Source: three-view drawing plus pictorial views. Frame: mm from the lowest corner of the part. A direction names the side the tool comes from. Round coordinates to 2 decimals unless told otherwise and drop trailing zeros. Loops run counter-clockwise (first coordinate to the right, second up) from the corner with the lowest first, then second, coordinate; pieces in that order, holes last. Notation, with made-up numbers: (2.25, 68.25) -> (32.25, 68.25) arc R8 ccw to (32.25, 80.25) -> close; hole circle Ø5 at (88, -34.75). An arc over 180 degrees is marked (long way). One line per question, with ' | ' between items. Start each with the question number.
Q1. Material intervals for L1, parallel to X at y = 1.25, z = 7.02; L2, parallel to X at y = 1, z = 1.94 (1 decimal); L3, parallel to X at y = 0.3, z = 2.75, sorted ascending.
Q2. Cut plane B-B on z = 8.75. Return loops of the section in (x, y).
Q3. Cut plane D-D on z = 5.75. Return loops of the section in (x, y).
Q4. Cut plane C-C on y = 1.15. Return loops of the section in (x, z), and give its area (3 significant figures).
Q5. Contact query for flat-ended pins moving along their axis: P1, Ø4, axis at x = 2.06, z = 8.75, coming from the -Y side; P2, Ø1, axis at x = 4.5, z = 3.5, coming from the +Y side. Output: stop coordinate, or through.
Q6. Cut plane A-A on x = 15. Return loops of the section in (y, z).
Q7. Mould query, pull axis X, two halves, no side actions, for the marked faces 1, 2 and 3. Classes: pulls with the +X half, pulls with the -X half, needs draft (parallel to the pull), parting line crosses it, or undercut.
Q8. Access query for the marked faces 4 and 5. Directions: +Z, -Z, +X, -X, +Y, -Y. A direction counts if a zero-diameter tool reaches every point of the face in a straight line with its end or side. Return the directions, or none.
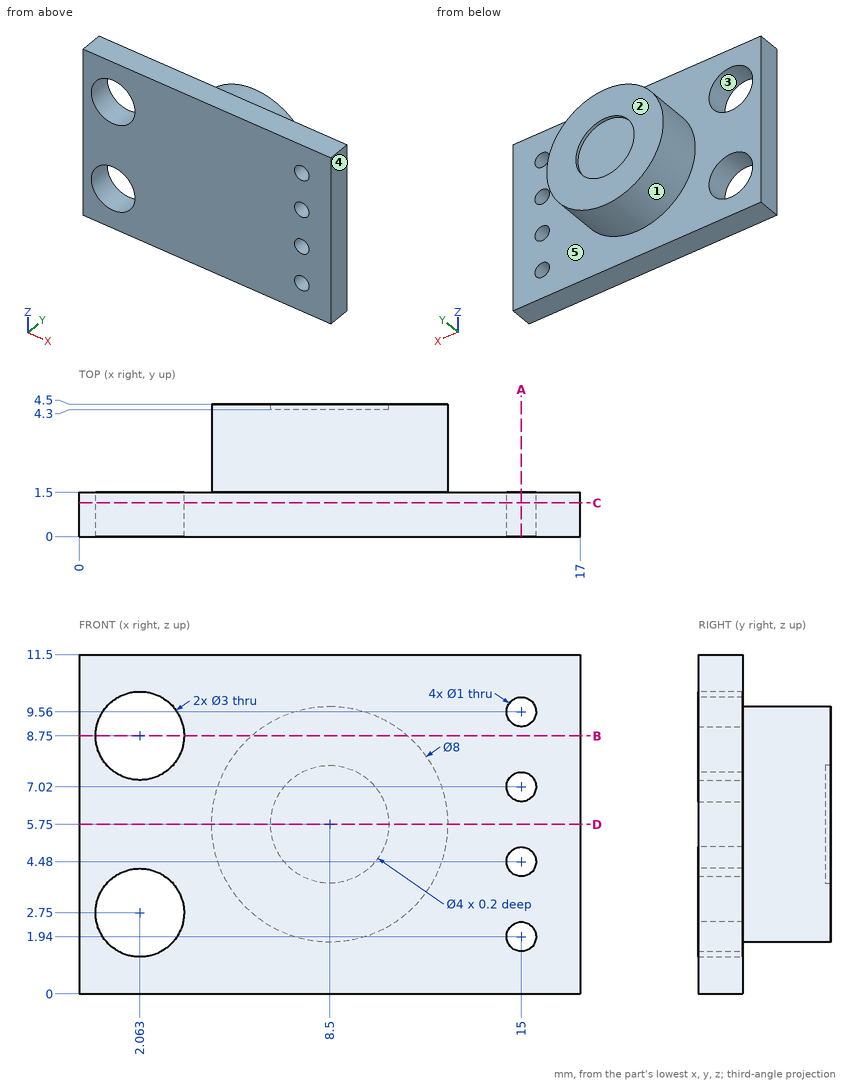
Results:
1) L1: 0 to 14.5, 15.5 to 17 | L2: 0 to 0.8, 3.3 to 14.5, 15.5 to 17 | L3: 0 to 0.56, 3.56 to 17
2) outline: (0, 0) -> (0.56, 0) -> (0.56, 1.5) -> (0, 1.5) -> close; (3.56, 0) -> (17, 0) -> (17, 1.5) -> (11.15, 1.5) -> (11.15, 4.5) -> (5.85, 4.5) -> (5.85, 1.5) -> (3.56, 1.5) -> close
3) outline: (0, 0) -> (17, 0) -> (17, 1.5) -> (12.5, 1.5) -> (12.5, 4.5) -> (10.5, 4.5) -> (10.5, 4.3) -> (6.5, 4.3) -> (6.5, 4.5) -> (4.5, 4.5) -> (4.5, 1.5) -> (0, 1.5) -> close
4) outline: (0, 0) -> (17, 0) -> (17, 11.5) -> (0, 11.5) -> close; hole circle Ø3 at (2.06, 2.75); hole circle Ø3 at (2.06, 8.75); hole circle Ø1 at (15, 1.94); hole circle Ø1 at (15, 4.48); hole circle Ø1 at (15, 7.02); hole circle Ø1 at (15, 9.56) | area: 178 mm^2
5) P1: y = 0 | P2: y = 1.5
6) outline: (0, 0) -> (1.5, 0) -> (1.5, 1.44) -> (0, 1.44) -> close; (0, 2.44) -> (1.5, 2.44) -> (1.5, 3.98) -> (0, 3.98) -> close; (0, 4.98) -> (1.5, 4.98) -> (1.5, 6.52) -> (0, 6.52) -> close; (0, 7.52) -> (1.5, 7.52) -> (1.5, 9.06) -> (0, 9.06) -> close; (0, 10.06) -> (1.5, 10.06) -> (1.5, 11.5) -> (0, 11.5) -> close
7) face 1: parting line crosses it | face 2: needs draft | face 3: undercut
8) face 4: +Z, -Z, +X, +Y, -Y | face 5: +Y
